```python
from build123d import *

# Parameters (mm, degrees)
F2_S5_R     = 16.67002
F2_T6_DEPTH = 26


# Not quite as in the source:
# - a fillet or chamfer that OpenCascade refuses, or shapes differently, is made with other operations: its cross-section is extruded or revolved along the edge and cut away or added


with BuildPart() as f1:
    # F0 (on Front) → F1 (revolve)
    with BuildSketch(Plane.XZ):
        Polygon((-17.7118646965, 0), (-16.1243646965, 1.5875), (-16.1243646965, 75.80376), (-16.67002, 75.80376), (-16.67002, 84.1375), (-18.25752, 84.1375), (-18.25752, 82.55), (-20.6375, 82.55), (-20.6375, 80.56626), (-18.2626, 80.56626), (-18.2626, 77.39126), (-20.6375, 77.39126), (-20.6375, 75.80376), (-19.05, 69.45376), (-19.05, 9.525), (-23.02002, 9.525), (-23.02002, 6.35), (-19.05, 6.35), (-19.05, 0), align=None)
    revolve(axis=Axis((0, 0, 38.1), (0, 0, 1)))

    # F2: chamfer of 0.8128 x 4.7625 on 1 edges, made by hand


with BuildPart() as f2_tool2:
    # F2_s3 → F2_t4 (revolve)
    with BuildSketch(Plane.XZ):
        Polygon((-16.1243646965, 71.04126), (-16.9371646965, 75.80376), (-16.1243646965, 75.80376), align=None)
    revolve(axis=Axis((0, 0, 75.80376), (0, 0, 1)))

    # F2_s5 → F2_t6 (intersect, symmetric)
    with BuildSketch(Plane.XY.offset(73.4)):
        Circle(F2_S5_R)
    extrude(amount=F2_T6_DEPTH, both=True, mode=Mode.INTERSECT)


with BuildPart() as f1_1:
    add(f1.part)

    # F2_t1: cut F2_tool2
    add(f2_tool2.part, mode=Mode.SUBTRACT)


solid = f1_1.part
```
Design review of the part built by this model. Coordinates are the model's own, in mm. A direction names the side the tool comes from. Give positions to 0.01 mm unless a question says otherwise; leave off trailing zeros. Write each loop counter-clockwise with the first axis right and the second up, starting at its lowest first coordinate (ties: lowest second). Pieces come first, ordered by that corner, then holes.
(1) Wall thickness on line 1 along Y through (x, z) = (0, 30); line 2 along Y through (x, z) = (0, 77.5): over which ranges is each line inside the solid? List them lowest first.
Checked values:
line 1: y = -19.05 to -16.12, 16.12 to 19.05
line 2: y = -18.26 to -16.67, 16.67 to 18.26
(2) Tool access review of faces 1 (the face through (4.474, 20.147, 81.544)), 2 (the face through (9, -17, 6.35)), 3 (the face through (-17.419, -5.486, 78.957)): name each direction out of +Z, -Z, +X, -X, +Y, -Y from which nothing blocks a thin tool from reaching the whole face with its end or side.
Checked values:
face 1: +Z
face 2: -Z
face 3: none
(3) Add section A-A (z = 17). Give the boundary of the cut face in (x, y), and give its area (3 significant figures).
Checked values:
outline: circle Ø38.1 at (0, 0); hole circle Ø32.25 at (0, 0)
area: 323 mm2
(4) Add section B-B (z = 7.5). Give the boundary of the cut face in (x, y), and give its area (3 significant figures).
Checked values:
outline: circle Ø46.04 at (0, 0); hole circle Ø32.25 at (0, 0)
area: 848 mm2
(5) Mouldability with a two-part tool opening along Z and no side actions: class faces 4 (the face through (-8, 17, 80.566)), 5 (the face through (8, 17, 82.55)), 6 (the face through (-9, -17, 9.525)), 7 (the face through (-15.38, -4.84, 36.8)) as +Z half, -Z half, draft (parallel to the pull), parting line (faces both ways), or undercut.
Checked values:
face 4: undercut
face 5: +Z half
face 6: undercut
face 7: draft
(6) Clearance check with flat-ended pins moving along their axes: pin 1 Ø12.5 at (x, y) = (-9, 4.5) entering from -Z; pin 2 Ø10 at (y, z) = (-6.5, 73) entering from +X; pin 3 Ø6 at (x, z) = (17.5, 54) entering from +Y. State where each tip first meets the part, or that it passes through.
Checked values:
pin 1: stops at z = 1.4
pin 2: stops at x = 20.5
pin 3: stops at y = 12.36
